The listing builds one solid part. Answer for the finished solid, in the listing's coordinates (mm). Face numbers are marked on the shaded views. A direction names the side the tool comes from. Give positions to 0.01 mm unless a question says otherwise; leave off trailing zeros. Loops run counter-clockwise (first coordinate to the right, second up) from the corner with the lowest first, then second, coordinate; pieces in that order, holes last. Notation, with made-up numbers: (45, -28) - (66, -28) arc R7 cw to (66, -17) - close; hole circle Ø10 at (72, 41.5). An arc over 180 degrees is marked (long way). One line per item, written item: value. Start each with the question number.
from build123d import *

# Parameters (mm, degrees)
F1_DEPTH = 61.976
F3_DEPTH = 35.814
F4_R     = 9.9949
F5_DEPTH = 42.926
F6_R     = 28.820882


with BuildPart() as f1:
    # F0 (on Top) → F1 (new body)
    with BuildSketch(Plane.XY):
        Polygon((-119.888, 0), (0, 0), (0, 19.9898), (-111.607954, 19.9898), (-176.33789, 84.719736), (-190.472813, 70.584813), align=None)
    extrude(amount=F1_DEPTH)

    # F2 (on face) → F3 (cut)
    with BuildSketch(Plane(origin=(0, 19.9898, 0), x_dir=(-1, 0, 0), z_dir=(0, 1, 0))):
        with BuildLine():
            Line((91.630854, 40.9829), (19.9771, 40.9829))
            ThreePointArc((19.9771, 40.9829), (9.9822, 30.988), (19.9771, 20.9931))
            Line((19.9771, 20.9931), (91.630854, 20.9931))
            ThreePointArc((91.630854, 20.9931), (101.625754, 30.988), (91.630854, 40.9829))
        make_face()
    extrude(amount=-F3_DEPTH, mode=Mode.SUBTRACT)

    # F4 (on face) → F5 (cut)
    with BuildSketch(Plane(origin=(-45.809077, -45.809077, 0), x_dir=(-0.707107, 0.707107, 0), z_dir=(0.707107, 0.707107, 0))):
        with Locations((164.618518, 30.988)):
            Circle(F4_R)
    extrude(amount=-F5_DEPTH, mode=Mode.SUBTRACT)

    # F6
    f6_edges = [f1.edges().sort_by_distance(p)[0] for p in [
        (-183.405352, 77.652275, 0),
        (-183.405352, 77.652275, 61.976),
    ]]
    fillet(f6_edges, radius=F6_R)


solid = f1.part
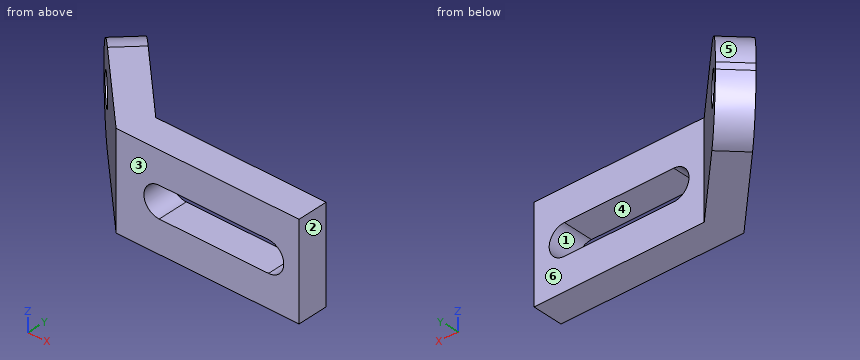
1. A cutting plane is placed at C-C (y = 13). Determine the outline of the cut face in (x, z), plus the area to 3 significant figures.
2. Flat-ended cylindrical pins translate along their axes: pin 1 (5 mm diameter, centred on x = -42.5, z = 50, fed in from +Y); pin 2 (12 mm diameter, centred on y = 55.5, z = 54.5, fed in from +X); pin 3 (1.5 mm diameter, centred on x = -143.5, z = 47.5, fed in from +Y). Find the tip coordinate at first contact, or state that the pin passes through.
3. Find the intervals of material crossed by L1, parallel to Z at x = -39, y = 16; L2, parallel to Y at x = -21, z = 56.5; L3, parallel to X at y = 16, z = 25, in increasing order. Write a range as [from, to].
4. A cutting plane is placed at B-B (z = 24). Determine the outline of the cut face in (x, y).
5. A cutting plane is placed at D-D (z = 11). Determine the outline of the cut face in (x, y) (3 decimals), plus the area to 3 significant figures.
6. Determine the mould class of the marked faces 1, 2 and 3 for opening direction X: released by +X, released by -X, zero draft, split by the parting line, or undercut.
7. For the marked faces 4, 5 and 6, determine the directions among +Z, -Z, +X, -X, +Y, -Y from which every point of the face is accessible in a straight line to the end or side of a thin tool.
8. A cutting plane is placed at A-A (x = -74.5). Determine the outline of the cut face in (y, z), plus the area to 3 significant figures.
Results below:
1. outline: (-132.89, 0) - (0, 0) - (0, 61.98) - (-132.89, 61.98) - close; hole (-91.63, 20.99) - (-19.98, 20.99) arc R9.99 ccw to (-19.98, 40.98) - (-91.63, 40.98) arc R9.99 ccw to start
1. area: 6,490 mm^2
2. pin 1: stops at y = 19.99
2. pin 2: stops at x = -141.12
2. pin 3: stops at y = 52.63
3. L1: z = [0, 20.99], [40.98, 61.98]
3. L2: y = [0, 19.99]
3. L3: x = [-135.89, -99.63], [-11.97, 0]
4. outline: (-190.19, 70.3) - (-181.4, 61.51) - (-167.26, 75.65) - (-176.05, 84.43) - close; (-171.29, 51.41) - (-119.89, 0) - (-98.78, 0) - (-98.78, 19.99) - (-111.61, 19.99) - (-157.16, 65.54) - close; (-12.83, 0) - (0, 0) - (0, 19.99) - (-12.83, 19.99) - close
5. outline: (-186.11, 66.222) - (-119.888, 0) - (0, 0) - (0, 19.99) - (-111.608, 19.99) - (-171.975, 80.357) - close
5. area: 4,100 mm^2
6. face 1: undercut
6. face 2: released by +X
6. face 3: zero draft
7. face 4: +Y, -Y
7. face 5: +Z, -X, +Y
7. face 6: +Z, -Z, +X, +Y
8. outline: (0, 0) - (19.99, 0) - (19.99, 20.99) - (0, 20.99) - close; (0, 40.98) - (19.99, 40.98) - (19.99, 61.98) - (0, 61.98) - close
8. area: 839 mm^2
